Geometry: final body of the model. Coordinates: model frame, mm. A direction names the side the tool comes from. Round coordinates to 2 decimals unless told otherwise and drop trailing zeros. Write each loop counter-clockwise with the first axis right and the second up, starting at its lowest first coordinate (ties: lowest second). Pieces come first, ordered by that corner, then holes. Notation, with made-up numbers: (81, 5.25) - (128, 5.25) arc R5 cw to (128, 13.25) - close; hole circle Ø5 at (69.5, 50.5). An arc over 180 degrees is marked (long way). Write each question's results on one line, items separated by ' | '.
from build123d import *

# Parameters (mm, degrees)
SKETCH1_W           = 40
SKETCH1_H           = 40
SKETCH1_R           = 19
BOSS_EXTRUDE1_DEPTH = 1
BOSS_EXTRUDE3_DEPTH = 40
CUT_EXTRUDE1_DEPTH  = 40
SKETCH4_W           = 2
SKETCH4_H           = 17.959199538
CUT_EXTRUDE2_DEPTH  = 40
SKETCH5_W           = 4.291289536
SKETCH5_H           = 2.060082618
BOSS_EXTRUDE4_DEPTH = 1
SKETCH6_W           = 40
SKETCH6_H           = 40.535957941
SKETCH6_R           = 19
BOSS_EXTRUDE5_DEPTH = 1
SKETCH7_W           = 2
SKETCH7_H           = 8.850816201
SKETCH7_H_2         = 7.048300719
BOSS_EXTRUDE6_DEPTH = 1
BOSS_EXTRUDE7_DEPTH = 40
SKETCH9_W           = 50
SKETCH9_H           = 50
BOSS_EXTRUDE8_DEPTH = 2
SKETCH10_R          = 23
CUT_EXTRUDE3_DEPTH  = 2


with BuildPart() as part:
    # Sketch1 → Boss-Extrude1 (new body)
    with BuildSketch(Plane(origin=(0, 0, 0), x_dir=(1, 0, 0), z_dir=(0, 1, 0))):
        with Locations((-20, -4.822405003)):
            Rectangle(SKETCH1_W, SKETCH1_H)
        with Locations((-20, -4.822405003)):
            Circle(SKETCH1_R, mode=Mode.SUBTRACT)
    extrude(amount=BOSS_EXTRUDE1_DEPTH)

    # Sketch2 → Boss-Extrude3 (add)
    with BuildSketch(Plane(origin=(0, 0, 0), x_dir=(0, 0, -1), z_dir=(1, 0, 0))):
        Polygon((15.177594997, 0), (26.251567878, -16.654342515), (27.084285004, -16.100643871), (15.713552938, 1), (15.177594997, 1), align=None)
    extrude(amount=-BOSS_EXTRUDE3_DEPTH)

    # Sketch3 → Cut-Extrude1 (cut)
    with BuildSketch(Plane(origin=(0, 6.997999648, -10.524414707), x_dir=(1, 0, 0), z_dir=(0, -0.553698644, 0.832717126))):
        Polygon((-20, -28.40381377), (-40, -8.40381377), (-40, -28.40381377), align=None)
    extrude(amount=-CUT_EXTRUDE1_DEPTH, mode=Mode.SUBTRACT)

    # Sketch4 → Cut-Extrude2 (cut)
    with BuildSketch(Plane(origin=(0, 6.997999648, -10.524414707), x_dir=(1, 0, 0), z_dir=(0, -0.553698644, 0.832717126))):
        with Locations((-5, -18.291545123)):
            Rectangle(SKETCH4_W, SKETCH4_H)
    extrude(amount=-CUT_EXTRUDE2_DEPTH, mode=Mode.SUBTRACT)

    # Sketch5 → Boss-Extrude4 (add)
    with BuildSketch(Plane(origin=(0, 6.997999648, -10.524414707), x_dir=(1, 0, 0), z_dir=(0, -0.553698644, 0.832717126))):
        with Locations((-5.191272024, -19.192802864)):
            Rectangle(SKETCH5_W, SKETCH5_H)
    extrude(amount=-BOSS_EXTRUDE4_DEPTH)

    # Sketch6 → Boss-Extrude5 (add)
    with BuildSketch(Plane(origin=(0, 1, 0), x_dir=(1, 0, 0), z_dir=(0, 1, 0))):
        with Locations((-20, -4.554426032)):
            Rectangle(SKETCH6_W, SKETCH6_H)
        with Locations((-20, -4.822405003)):
            Circle(SKETCH6_R, mode=Mode.SUBTRACT)
    extrude(amount=BOSS_EXTRUDE5_DEPTH)

    # Sketch7 → Boss-Extrude6 (add)
    with BuildSketch(Plane(origin=(0, 7.551698292, -11.357131833), x_dir=(-1, 0, 0), z_dir=(0, 0.553698644, -0.832717126))):
        Polygon((40, -7.867855829), (40, -8.40381377), (20, -28.40381377), (0, -28.40381377), (0, -7.867855829), align=None)
        with Locations((5, -13.737353454)):
            Rectangle(SKETCH7_W, SKETCH7_H, mode=Mode.SUBTRACT)
        with Locations((5, -23.746994533)):
            Rectangle(SKETCH7_W, SKETCH7_H_2, mode=Mode.SUBTRACT)
    extrude(amount=BOSS_EXTRUDE6_DEPTH)

    # Sketch8 → Boss-Extrude7 (add)
    with BuildSketch(Plane(origin=(0, 0, 0), x_dir=(0, 0, -1), z_dir=(1, 0, 0))):
        Polygon((15.713552938, 2), (16.546270063, 1.553698644), (15.713552938, 1), align=None)
    extrude(amount=-BOSS_EXTRUDE7_DEPTH)

    # Sketch9 → Boss-Extrude8 (add)
    with BuildSketch(Plane(origin=(0, 0, 0), x_dir=(-1, 0, 0), z_dir=(0, -1, 0))):
        with Locations((25, -9.822405003)):
            Rectangle(SKETCH9_W, SKETCH9_H)
    extrude(amount=-BOSS_EXTRUDE8_DEPTH)

    # Sketch10 → Cut-Extrude3 (cut)
    with BuildSketch(Plane(origin=(0, 0, 0), x_dir=(-1, 0, 0), z_dir=(0, -1, 0))):
        with Locations((25, -9.822405003)):
            Circle(SKETCH10_R)
    extrude(amount=-CUT_EXTRUDE3_DEPTH, mode=Mode.SUBTRACT)


solid = part.part
Q1. Section query B-B, the plane z = 24. Return loops of the section in (x, y), plus the area to 3 significant figures.
Answer block:
outline: (-50, 0) - (-43.11, 0) - (-43.11, 2) - (-50, 2) - close; (-6.89, 0) - (0, 0) - (0, 2) - (-6.89, 2) - close | area: 27.6 mm2
Q2. Pin query (flat end, axial travel): pin 1 (4.5 mm diameter, centred on y = -10.5, z = -23.5, fed in from -X); pin 2 (1.5 mm diameter, centred on x = -39.5, z = -17.5, fed in from +Y); pin 3 (6 mm diameter, centred on x = -35.5, y = -4, fed in from +Z). Return the tip coordinate at first contact, or that it passes through.
Answer block:
pin 1: x = -28.9 | pin 2: y = 1.25 | pin 3: z = -15.84
Q3. Section query A-A, the plane x = -25. Return loops of the section in (y, z), plus the area to 3 significant figures.
Answer block:
outline: (-12.49, -23.48) - (-11.38, -25.15) - (1.55, -16.55) - (2, -15.71) - (2, -13.18) - (0, -13.18) - (0, -15.18) - close; (0, 32.82) - (2, 32.82) - (2, 34.82) - (0, 34.82) - close | area: 40.0 mm2
Q4. Ray query, line 1 along Z through (x, y) = (-25, 1.55); line 2 along Z through (x, y) = (-25, 1.4); line 3 along X through (y, z) = (0.25, 19.5). Return the intervals inside material, ascending.
Answer block:
line 1: -16.55 to -13.18, 32.82 to 34.82 | line 2: -16.65 to -13.18, 32.82 to 34.82 | line 3: -50 to -45.86, -4.14 to 0
Q5. Section query D-D, the plane x = -16.5. Return loops of the section in (y, z).
Answer block:
outline: (-16.65, -26.25) - (-15.55, -27.92) - (1.55, -16.55) - (2, -15.71) - (2, -11.55) - (0, -11.55) - (0, -15.18) - close; (0, 31.19) - (2, 31.19) - (2, 34.82) - (0, 34.82) - close
Q6. Access query for faces 1 (the flat face through (-4.99, -9.3, -22.54)), 2 (the flat face through (-15.836, -6.877, -22.152)), 3 (the flat face through (-4.99, -7.58, -21.4)), 4 (the flat face through (-45, 1, -15.178)), 5 (the flat face through (-4.5, 0, -1.4)). Directions: +Z, -Z, +X, -X, +Y, -Y. A direction counts if a zero-diameter tool reaches every point of the face in a straight line with its end or side. Return the directions, or none.
Answer block:
face 1: -Z, -Y | face 2: -Z, +X, -X, +Y | face 3: +Z, +Y | face 4: -Z, -X, +Y, -Y | face 5: +Z, +X, -X, -Y
Q7. Section query C-C, the plane y = -3.5. Return loops of the section in (x, z).
Answer block:
outline: (-35.8, -17.5) - (-34.47, -19.91) - (-6, -19.91) - (-6, -17.5) - close; (-4, -19.91) - (0, -19.91) - (0, -17.5) - (-4, -17.5) - close
Q8. Mould query, pull axis Z, two halves, no side actions, for faces 6 (the flat face through (-4.986, -15.165, -26.445)), 7 (the flat face through (-30.14, -7.66, -21.46)), 8 (the cylindrical face through (-6.75, 0.99, 23.82)), 9 (the flat face through (-40, 1, -16)). Classes: pulls with the +Z half, pulls with the -Z half, needs draft (parallel to the pull), parting line crosses it, or undercut.
Answer block:
face 6: pulls with the +Z half | face 7: pulls with the -Z half | face 8: undercut | face 9: needs draft
